Could you check a few things on this model? Use its own coordinates, in mm. Face numbers are marked on the shaded views. Give positions to 0.01 mm unless a question says otherwise; leave off trailing zeros. Order: outer loops, then holes, each group sorted by start corner. A loop starts at its lowest first (then second) coordinate and runs counter-clockwise, first axis right, second up.
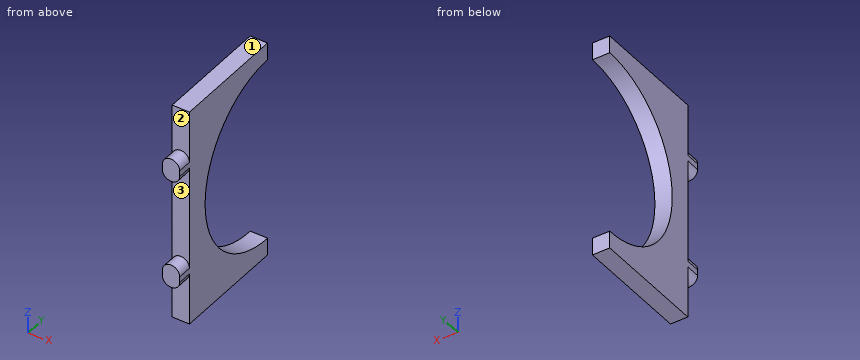
from build123d import *

# Parameters (mm, degrees)
BOSS_EXTRUDE1_DEPTH = 6
BOSS_EXTRUDE2_DEPTH = 5


with BuildPart() as part:
    # Sketch1 → Boss-Extrude1 (new body)
    with BuildSketch(Plane(origin=(0, 0, 0), x_dir=(0, 0, -1), z_dir=(1, 0, 0))):
        with BuildLine():
            Line((-38, 0), (-32, 0))
            ThreePointArc((-32, 0), (0, -32), (32, 0))
            Line((32, 0), (38, 0))
            Line((38, 0), (38, -40))
            Line((38, -40), (-38, -40))
            Line((-38, -40), (-38, 0))
        make_face()
    extrude(amount=BOSS_EXTRUDE1_DEPTH)

    # Sketch3 → Boss-Extrude2 (add)
    with BuildSketch(Plane.XZ.offset(40)):
        with BuildLine():
            Line((0, 20), (0, 18))
            ThreePointArc((0, 18), (3, 15), (6, 18))
            Line((6, 18), (6, 20))
            ThreePointArc((6, 20), (3, 23), (0, 20))
        make_face()
        with BuildLine():
            Line((0, -18), (0, -20))
            ThreePointArc((0, -20), (3, -23), (6, -20))
            Line((6, -20), (6, -18))
            ThreePointArc((6, -18), (3, -15), (0, -18))
        make_face()
    extrude(amount=BOSS_EXTRUDE2_DEPTH)


solid = part.part
Item 1: Imagine slicing it at B-B on x = 3. List the corners of the cut face in (y, z) for me.
Findings:
outline: (-45, -23) - (-40, -23) - (-40, -38) - (0, -38) - (0, -32) arc R32 cw to (0, 32) - (0, 38) - (-40, 38) - (-40, 23) - (-45, 23) - (-45, 15) - (-40, 15) - (-40, -15) - (-45, -15) - close
Item 2: Imagine slicing it at A-A on y = -23. List the corners of the cut face in (x, z) for me.
Findings:
outline: (0, -38) - (6, -38) - (6, -22.25) - (0, -22.25) - close; (0, 22.25) - (6, 22.25) - (6, 38) - (0, 38) - close
Item 3: Imagine slicing it at D-D on y = -28. List the corners of the cut face in (x, z) for me, then the cut area to 3 significant figures.
Findings:
outline: (0, -38) - (6, -38) - (6, -15.49) - (0, -15.49) - close; (0, 15.49) - (6, 15.49) - (6, 38) - (0, 38) - close
area: 270 mm2
Item 4: Please list where these lines run through material, in increasing order: line 1 along Z through (x, y) = (2.3, -40.5); line 2 along Z through (x, y) = (5.2, -19.5); line 3 along Y through (x, z) = (4.4, -11).
Findings:
line 1: z = -22.92 to -15.08, 15.08 to 22.92
line 2: z = -38 to -25.37, 25.37 to 38
line 3: y = -40 to -30.05
Item 5: Imagine slicing it at C-C on z = 0. List the corners of the cut face in (x, y) for me.
Findings:
outline: (0, -40) - (6, -40) - (6, -32) - (0, -32) - close
Item 6: We'd pull the mould along Z, two halves only. Please class the marked faces 1, 2 and 3: +Z half, -Z half, draft (parallel to the pull), parting line (faces both ways), or undercut.
Findings:
face 1: +Z half
face 2: draft
face 3: undercut
Item 7: For pin 1 (1.8 mm diameter, centred on x = 4, z = -30, fed in from -Y); pin 2 (6 mm diameter, centred on y = -32.5, z = -4, fed in from -X); pin 3 (8 mm diameter, centred on y = -24, z = -3, fed in from -X), each with a flat end and sliding along its axis, tell me the tip position at first contact or that it passes through.
Findings:
pin 1: stops at y = -40
pin 2: stops at x = 0
pin 3: passes through
